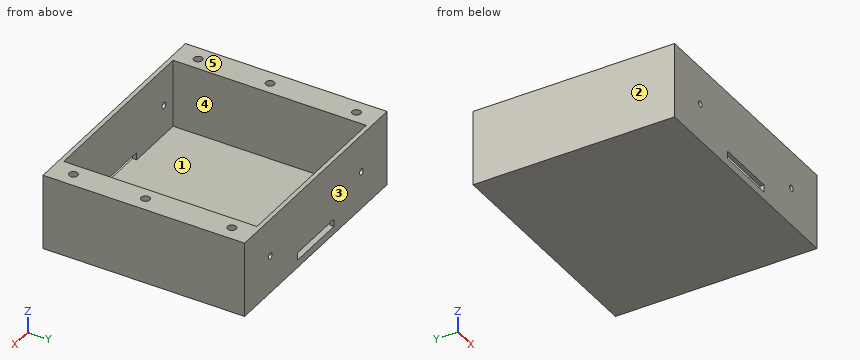
from build123d import *

# Parameters (mm, degrees)
F0_W     = 146.05
F0_H     = 133.35
F0_R     = 3.24
F0_W_2   = 5
F1_DEPTH = 50
F2_D     = 5.6
F2_DEPTH = 20
F2_TIP   = 1.6824097333
F3_W     = 119.824
F3_H     = 127.75
F4_DEPTH = 45
F5_W     = 40
F5_H     = 5
F6_DEPTH = 133.351
F7_D     = 4


with BuildPart() as f1:
    # F0 (on Top) → F1 (new body)
    with BuildSketch(Plane.XY):
        Rectangle(F0_W, F0_H)
        with Locations((-68.262, -52.387)):
            Circle(F0_R, mode=Mode.SUBTRACT)
        with Locations((-68.262, -4.7625)):
            Circle(F0_R, mode=Mode.SUBTRACT)
        with Locations((68.262, -52.387)):
            Circle(F0_R, mode=Mode.SUBTRACT)
        with Locations((68.262, -4.7625)):
            Circle(F0_R, mode=Mode.SUBTRACT)
        with BuildLine():
            Line((72.225, 46.037), (72.225, 1.5875))
            Line((72.225, 1.5875), (68.262, 1.5875))
            ThreePointArc((68.262, 1.5875), (61.912, -4.7625), (68.262, -11.1125))
            Line((68.262, -11.1125), (72.225, -11.1125))
            Line((72.225, -11.1125), (72.225, -46.037))
            Line((72.225, -46.037), (68.262, -46.037))
            ThreePointArc((68.262, -46.037), (61.912, -52.387), (68.262, -58.737))
            Line((68.262, -58.737), (72.225, -58.737))
            Line((72.225, -58.737), (72.225, -65.875))
            Line((72.225, -65.875), (-72.225, -65.875))
            Line((-72.225, -65.875), (-72.225, -58.737))
            Line((-72.225, -58.737), (-68.262, -58.737))
            ThreePointArc((-68.262, -58.737), (-61.912, -52.387), (-68.262, -46.037))
            Line((-68.262, -46.037), (-72.225, -46.037))
            Line((-72.225, -46.037), (-72.225, -11.1125))
            Line((-72.225, -11.1125), (-68.262, -11.1125))
            ThreePointArc((-68.262, -11.1125), (-61.912, -4.7625), (-68.262, 1.5875))
            Line((-68.262, 1.5875), (-72.225, 1.5875))
            Line((-72.225, 1.5875), (-72.225, 46.037))
            Line((-72.225, 46.037), (-68.262, 46.037))
            ThreePointArc((-68.262, 46.037), (-61.912, 52.387), (-68.262, 58.737))
            Line((-68.262, 58.737), (-72.225, 58.737))
            Line((-72.225, 58.737), (-72.225, 65.875))
            Line((-72.225, 65.875), (72.225, 65.875))
            Line((72.225, 65.875), (72.225, 58.737))
            Line((72.225, 58.737), (68.262, 58.737))
            ThreePointArc((68.262, 58.737), (61.912, 52.387), (68.262, 46.037))
            Line((68.262, 46.037), (72.225, 46.037))
        make_face(mode=Mode.SUBTRACT)
        with Locations((-68.262, 52.387)):
            Circle(F0_R, mode=Mode.SUBTRACT)
        with Locations((68.262, 52.387)):
            Circle(F0_R, mode=Mode.SUBTRACT)
        with BuildLine():
            Line((68.262, 1.5875), (72.225, 1.5875))
            Line((72.225, 1.5875), (72.225, 46.037))
            Line((72.225, 46.037), (68.262, 46.037))
            ThreePointArc((68.262, 46.037), (61.912, 52.387), (68.262, 58.737))
            Line((68.262, 58.737), (72.225, 58.737))
            Line((72.225, 58.737), (72.225, 65.875))
            Line((72.225, 65.875), (-72.225, 65.875))
            Line((-72.225, 65.875), (-72.225, 58.737))
            Line((-72.225, 58.737), (-68.262, 58.737))
            ThreePointArc((-68.262, 58.737), (-61.912, 52.387), (-68.262, 46.037))
            Line((-68.262, 46.037), (-72.225, 46.037))
            Line((-72.225, 46.037), (-72.225, 1.5875))
            Line((-72.225, 1.5875), (-68.262, 1.5875))
            ThreePointArc((-68.262, 1.5875), (-61.912, -4.7625), (-68.262, -11.1125))
            Line((-68.262, -11.1125), (-72.225, -11.1125))
            Line((-72.225, -11.1125), (-72.225, -46.037))
            Line((-72.225, -46.037), (-68.262, -46.037))
            ThreePointArc((-68.262, -46.037), (-61.912, -52.387), (-68.262, -58.737))
            Line((-68.262, -58.737), (-72.225, -58.737))
            Line((-72.225, -58.737), (-72.225, -65.875))
            Line((-72.225, -65.875), (72.225, -65.875))
            Line((72.225, -65.875), (72.225, -58.737))
            Line((72.225, -58.737), (68.262, -58.737))
            ThreePointArc((68.262, -58.737), (61.912, -52.387), (68.262, -46.037))
            Line((68.262, -46.037), (72.225, -46.037))
            Line((72.225, -46.037), (72.225, -11.1125))
            Line((72.225, -11.1125), (68.262, -11.1125))
            ThreePointArc((68.262, -11.1125), (61.912, -4.7625), (68.262, 1.5875))
        make_face()
        with Locations((-75.525, 0)):
            Rectangle(F0_W_2, F0_H)
        with Locations((75.525, 0)):
            Rectangle(F0_W_2, F0_H)
        with Locations((-68.262, 52.387)):
            Circle(F0_R)
        with Locations((-68.262, -4.7625)):
            Circle(F0_R)
        with Locations((-68.262, -52.387)):
            Circle(F0_R)
        with Locations((68.262, -52.387)):
            Circle(F0_R)
        with Locations((68.262, -4.7625)):
            Circle(F0_R)
        with Locations((68.262, 52.387)):
            Circle(F0_R)
    extrude(amount=-F1_DEPTH)

    # F2
    with Locations(Plane.XY):
        with Locations((-68.262, 52.387), (-68.262, -4.7625), (-68.262, -52.387), (68.262, -52.387), (68.262, -4.7625), (68.262, 52.387)):
            Hole(F2_D / 2, depth=F2_DEPTH)
            with Locations((0, 0, -(F2_DEPTH + F2_TIP / 2))):  # 118° drill point
                Cone(0, F2_D / 2, F2_TIP, mode=Mode.SUBTRACT)

    # F3 (on face) → F4 (cut)
    with BuildSketch(Plane.XY):
        Rectangle(F3_W, F3_H)
    extrude(amount=-F4_DEPTH, mode=Mode.SUBTRACT)

    # F5 (on face) → F6 (cut, through all)
    with BuildSketch(Plane.XZ.offset(66.675)):
        with Locations((0, -42.5)):
            Rectangle(F5_W, F5_H)
    extrude(amount=-F6_DEPTH, mode=Mode.SUBTRACT)

    # F7 (through all)
    with Locations(Plane.XZ.offset(66.675)):
        with Locations((-49.912, -25), (49.912, -25)):
            Hole(F7_D / 2)


solid = f1.part
Verification items for the finished model (mm, model axes). Face numbers are marked on the shaded views. A direction names the side the tool comes from. Round coordinates to 2 decimals unless told otherwise and drop trailing zeros. Loops run counter-clockwise (first coordinate to the right, second up) from the corner with the lowest first, then second, coordinate; pieces in that order, holes last. Notation, with made-up numbers: (-21, 81) - (27, 81) arc R10 cw to (27, 91) - close; hole circle Ø2 at (18.5, -18). An arc over 180 degrees is marked (long way). Use a Markdown table: item, result. Add a question column.
1. Release check for a two-part mould opening along Y. For the marked faces 1, 2 and 3 record: released by +Y, released by -Y, zero draft, split by the parting line, or undercut.
2. Section check D-D, the plane z = -12. Record the boundary of the cut face in (x, y) (1 decimal), plus the area to 3 significant figures.
3. Thickness scan on probe 1 along Y at (x, z) = (32.5, -35) (3 decimals); probe 2 along X at (y, z) = (31.5, -7.5) (3 decimals); probe 3 along Y at (x, z) = (66.5, -16.5) (3 decimals). Record the ranges inside material, lowest first. Write a range as [from, to].
4. Access from +Z, -Z, +X, -X, +Y, -Y to the whole of each face (thin tool, end or side, straight path). Record for the marked faces 4 and 5.
5. Section check B-B, the plane y = 24.5. Record the boundary of the cut face in (x, z) (3 decimals).
6. Gauge pin test, flat ends, axial feed: pin 1 (3.5 mm diameter, centred on x = -68.262, y = 52.387, fed in from +Z); pin 2 (5 mm diameter, centred on x = 68.26, y = -4.76, fed in from +Z); pin 3 (4 mm diameter, centred on x = 53.5, y = 10, fed in from +Z). Record the tip position at first contact, or that the pin passes through.
7. Section check A-A, the plane x = 3. Record the boundary of the cut face in (y, z) (3 decimals), plus the area to 3 significant figures.
8. Section check C-C, the plane z = -25. Record the boundary of the cut face in (x, y) (3 decimals), plus the area to 3 significant figures.
Checks:
| question | item | result |
|---|---|---|
| 1 | face 1 | undercut |
| 1 | face 2 | zero draft |
| 1 | face 3 | released by +Y |
| 2 | outline | (-78, -66.7) - (78, -66.7) - (78, 66.7) - (-78, 66.7) - close; hole circle Ø5.6 at (-68.3, -52.4); hole circle Ø5.6 at (-68.3, -4.8); hole circle Ø5.6 at (-68.3, 52.4); hole (-59.9, -63.9) - (59.9, -63.9) - (59.9, 63.9) - (-59.9, 63.9) - close; hole circle Ø5.6 at (68.3, -52.4); hole circle Ø5.6 at (68.3, -4.8); hole circle Ø5.6 at (68.3, 52.4) |
| 2 | area | 5,350 mm^2 |
| 3 | probe 1 | y = [-66.675, -63.875], [63.875, 66.675] |
| 3 | probe 2 | x = [-78.025, -59.912], [59.912, 78.025] |
| 3 | probe 3 | y = [-66.675, -54.563], [-50.211, -6.939], [-2.586, 50.211], [54.563, 66.675] |
| 4 | face 4 | +Z |
| 4 | face 5 | +Z, +X, -X, +Y, -Y |
| 5 | outline | (-78.025, -50) - (78.025, -50) - (78.025, 0) - (59.912, 0) - (59.912, -45) - (-59.912, -45) - (-59.912, 0) - (-78.025, 0) - close |
| 6 | pin 1 | stops at z = -20.63 |
| 6 | pin 2 | stops at z = -20.18 |
| 6 | pin 3 | stops at z = -45 |
| 7 | outline | (-66.675, -50) - (66.675, -50) - (66.675, -45) - (-66.675, -45) - close; (-66.675, -40) - (-63.875, -40) - (-63.875, 0) - (-66.675, 0) - close; (63.875, -40) - (66.675, -40) - (66.675, 0) - (63.875, 0) - close |
| 7 | area | 891 mm^2 |
| 8 | outline | (-78.025, -66.675) - (-51.912, -66.675) - (-51.912, -63.875) - (-59.912, -63.875) - (-59.912, 63.875) - (-51.912, 63.875) - (-51.912, 66.675) - (-78.025, 66.675) - close; (-47.912, -66.675) - (47.912, -66.675) - (47.912, -63.875) - (-47.912, -63.875) - close; (-47.912, 63.875) - (47.912, 63.875) - (47.912, 66.675) - (-47.912, 66.675) - close; (51.912, -66.675) - (78.025, -66.675) - (78.025, 66.675) - (51.912, 66.675) - (51.912, 63.875) - (59.912, 63.875) - (59.912, -63.875) - (51.912, -63.875) - close |
| 8 | area | 5,460 mm^2 |
